For this review, take the finished solid that the model builds, in its own axes (mm). Face numbers are marked on the shaded views. A direction names the side the tool comes from. Give positions to 0.01 mm unless a question says otherwise; leave off trailing zeros. Loops run counter-clockwise (first coordinate to the right, second up) from the corner with the lowest first, then second, coordinate; pieces in that order, holes last.
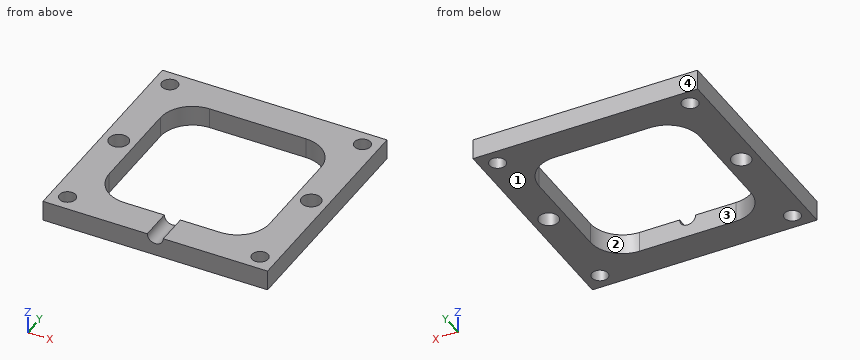
```python
from build123d import *

# Parameters (mm, degrees)
F1_DEPTH = 6.35
F3_D     = 5
F3_DEPTH = 14.4
F3_TIP   = 1.5021515476
F5_D     = 5
F5_DEPTH = 15
F5_TIP   = 1.5021515476


with BuildPart() as f1:
    # F0 (on Top) → F1 (new body)
    with BuildSketch(Plane.XY):
        with BuildLine():
            Line((-35, -35), (35, -35))
            Line((35, -35), (35, 0))
            Line((35, 0), (33, 0))
            ThreePointArc((33, 0), (30, -3), (27, 0))
            Line((27, 0), (25, 0))
            Line((25, 0), (25, -15))
            ThreePointArc((25, -15), (22.0710678119, -22.0710678119), (15, -25))
            Line((15, -25), (-15, -25))
            ThreePointArc((-15, -25), (-22.0710678119, -22.0710678119), (-25, -15))
            Line((-25, -15), (-25, 0))
            Line((-25, 0), (-27, 0))
            ThreePointArc((-27, 0), (-30, -3), (-33, 0))
            Line((-33, 0), (-35, 0))
            Line((-35, 0), (-35, -35))
        make_face()
        with BuildLine():
            Line((33, 0), (35, 0))
            Line((35, 0), (35, 35))
            Line((35, 35), (-35, 35))
            Line((-35, 35), (-35, 0))
            Line((-35, 0), (-33, 0))
            ThreePointArc((-33, 0), (-30, 3), (-27, 0))
            Line((-27, 0), (-25, 0))
            Line((-25, 0), (-25, 15))
            ThreePointArc((-25, 15), (-22.0710678119, 22.0710678119), (-15, 25))
            Line((-15, 25), (15, 25))
            ThreePointArc((15, 25), (22.0710678119, 22.0710678119), (25, 15))
            Line((25, 15), (25, 0))
            Line((25, 0), (27, 0))
            ThreePointArc((27, 0), (30, 3), (33, 0))
        make_face()
    extrude(amount=F1_DEPTH)

    # F3
    with Locations(Plane.XZ.offset(35)):
        with Locations((0, 6.35)):
            Hole(F3_D / 2, depth=F3_DEPTH)
            with Locations((0, 0, -(F3_DEPTH + F3_TIP / 2))):  # 118° drill point
                Cone(0, F3_D / 2, F3_TIP, mode=Mode.SUBTRACT)

    # F5
    with Locations(Plane(origin=(0, 0, 0), x_dir=(1, 0, 0), z_dir=(0, 0, -1))):
        with Locations((-30, 30), (30, 30), (30, -30), (-30, -30)):
            Hole(F5_D / 2, depth=F5_DEPTH)
            with Locations((0, 0, -(F5_DEPTH + F5_TIP / 2))):  # 118° drill point
                Cone(0, F5_D / 2, F5_TIP, mode=Mode.SUBTRACT)


solid = f1.part
```
Item 1: Clearance check with a flat-ended pin moving along its axis: pin 1 Ø4.5 at (x, y) = (30, 30) entering from +Z. State where the tip first meets the part, or that it passes through.
Answer:
pin 1: passes through
Item 2: Take a section at A-A on x = -30. Give the boundary of the cut face in (y, z), and give its area (3 significant figures).
Answer:
outline: (-35, 0) - (-32.5, 0) - (-32.5, 6.35) - (-35, 6.35) - close; (-27.5, 0) - (-3, 0) - (-3, 6.35) - (-27.5, 6.35) - close; (3, 0) - (27.5, 0) - (27.5, 6.35) - (3, 6.35) - close; (32.5, 0) - (35, 0) - (35, 6.35) - (32.5, 6.35) - close
area: 343 mm2
Item 3: Take a section at D-D on z = 2.25. Give the boundary of the cut face in (x, y), and give its area (3 significant figures).
Answer:
outline: (-35, -35) - (35, -35) - (35, 35) - (-35, 35) - close; hole circle Ø6 at (-30, 0); hole circle Ø5 at (-30, -30); hole circle Ø5 at (-30, 30); hole (-25, -15) arc R10 ccw to (-15, -25) - (15, -25) arc R10 ccw to (25, -15) - (25, 15) arc R10 ccw to (15, 25) - (-15, 25) arc R10 ccw to (-25, 15) - close; hole circle Ø6 at (30, 0); hole circle Ø5 at (30, -30); hole circle Ø5 at (30, 30)
area: 2,350 mm2
Item 4: Take a section at C-C on y = 0. Give the boundary of the cut face in (x, z), and give its area (3 significant figures).
Answer:
outline: (-35, 0) - (-33, 0) - (-33, 6.35) - (-35, 6.35) - close; (-27, 0) - (-25, 0) - (-25, 6.35) - (-27, 6.35) - close; (25, 0) - (27, 0) - (27, 6.35) - (25, 6.35) - close; (33, 0) - (35, 0) - (35, 6.35) - (33, 6.35) - close
area: 50.8 mm2
Item 5: The part is to be moulded in two halves that separate along X. For the marked faces 3 and 4, say which applies: released by +X, released by -X, zero draft, split by the parting line, or undercut.
Answer:
face 3: undercut
face 4: zero draft
Item 6: Take a section at B-B on y = -30. Give the boundary of the cut face in (x, z), and give its area (3 significant figures).
Answer:
outline: (-35, 0) - (-32.5, 0) - (-32.5, 6.35) - (-35, 6.35) - close; (-27.5, 0) - (27.5, 0) - (27.5, 6.35) - (2.5, 6.35) arc R2.5 cw to (-2.5, 6.35) - (-27.5, 6.35) - close; (32.5, 0) - (35, 0) - (35, 6.35) - (32.5, 6.35) - close
area: 371 mm2
Item 7: Tool access review of the marked faces 1 and 2: name each direction out of +Z, -Z, +X, -X, +Y, -Y from which nothing blocks a thin tool from reaching the whole face with its end or side.
Answer:
face 1: -Z, +X, -X, +Y, -Y
face 2: +Z, -Z
Item 8: For L1, parallel to X at y = 30, z = 4.75; L2, parallel to Y at x = 4, z = 2; L3, parallel to X at y = 30.5, z = 5.5, list the stretches that pass through material, from the lowest coordinate up.
Answer:
L1: x = -35 to -32.5, -27.5 to 27.5, 32.5 to 35
L2: y = -35 to -25, 25 to 35
L3: x = -35 to -32.45, -27.55 to 27.55, 32.45 to 35
